Work out the finished part from the listing and answer in its coordinate system (mm). A direction names the side the tool comes from. Round coordinates to 2 decimals unless told otherwise and drop trailing zeros. Loops run counter-clockwise (first coordinate to the right, second up) from the corner with the lowest first, then second, coordinate; pieces in that order, holes last. Notation, with made-up numbers: (8.5, 74.5) - (65.5, 74.5) arc R27 cw to (65.5, 104.5) - close; hole circle Ø7 at (43, 26). An arc over 180 degrees is marked (long way). Use CSV: the item, a comma, the result in double quotes. Start each with the question number.
from build123d import *

# Parameters (mm, degrees)
EXTRUDE1_DEPTH      = 4
EXTRUDE2_DEPTH      = 12.357816692
EXTRUDE2_DEPTH_BACK = 12.357816692
SKETCH2_R           = 1
EXTRUDE3_DEPTH      = 12.357816692
EXTRUDE3_DEPTH_BACK = 12.357816692
SKETCH4_W           = 6
SKETCH4_H           = 8.732029078
FILLET1_R           = 0.2
FILLET2_R           = 1
EXTRUDE4_DEPTH      = 14
EXTRUDE4_DEPTH_BACK = 3
SKETCH3_R           = 1.5
EXTRUDE5_DEPTH      = 9
SKETCH6_R           = 1.5
EXTRUDE6_DEPTH      = 1
SKETCH7_R           = 0.6
EXTRUDE7_DEPTH      = 1
FILLET3_R           = 1
SKETCH8_R           = 2
EXTRUDE8_DEPTH      = 1
SKETCH9_W           = 5.922368331
SKETCH9_H           = 2.817570744
SKETCH9_H_2         = 4.117351233
EXTRUDE9_DEPTH      = 19.227726134


with BuildPart() as part:
    # Sketch1 → Extrude1 (new, symmetric)
    with BuildSketch(Plane.XY):
        Polygon((0, 0), (-7, 0), (-7, 8), (7, 8), (7, 0), align=None)
    extrude(amount=EXTRUDE1_DEPTH, both=True)

    # Sketch2 → Extrude2 (cut, two sides: drawn at the far end of the back side and taken through both)
    with BuildSketch(Plane.XY.offset(-EXTRUDE2_DEPTH_BACK)):
        with Locations((4.5, 4.5)):
            Circle(SKETCH2_R)
    extrude(amount=EXTRUDE2_DEPTH + EXTRUDE2_DEPTH_BACK, mode=Mode.SUBTRACT)

    # Sketch4 → Extrude3 (cut, two sides: drawn at the far end of the back side and taken through both)
    with BuildSketch(Plane(origin=(0, 0, 0), x_dir=(0, 0, -1), z_dir=(1, 0, 0)).offset(-EXTRUDE3_DEPTH_BACK)):
        with Locations((0, 5.366014539)):
            Rectangle(SKETCH4_W, SKETCH4_H)
    extrude(amount=EXTRUDE3_DEPTH + EXTRUDE3_DEPTH_BACK, mode=Mode.SUBTRACT)

    # Fillet1
    fillet1_edges = [part.edges().sort_by_distance(p)[0] for p in [
        (0, 0, 4),
        (0, 0, -4),
    ]]
    fillet(fillet1_edges, radius=FILLET1_R)

    # Fillet2
    fillet2_edges = [part.edges().sort_by_distance(p)[0] for p in [
        (-7, 8, -3.5),
        (7, 8, -3.5),
        (-7, 8, 3.5),
        (7, 8, 3.5),
    ]]
    fillet(fillet2_edges, radius=FILLET2_R)

    # Sketch3 → Extrude4 (add, two sides: drawn at the far end of the back side and taken through both)
    with BuildSketch(Plane.XY.offset(-EXTRUDE4_DEPTH_BACK)):
        with Locations((-3, 4.5)):
            Circle(SKETCH3_R)
    extrude(amount=EXTRUDE4_DEPTH + EXTRUDE4_DEPTH_BACK)

    # Sketch5 → Extrude5 (cut)
    with BuildSketch(Plane.XY.offset(14)):
        Polygon((-4, 4.5), (-4, 6.060686456), (-4.95644391, 6.060686456), (-4.95644391, 2.5), (-4, 2.5), align=None)
    extrude(amount=-EXTRUDE5_DEPTH, mode=Mode.SUBTRACT)

    # Sketch6 → Extrude6 (add)
    with BuildSketch(Plane.XZ):
        with Locations((-7, 0)):
            Circle(SKETCH6_R)
        with Locations((7, 0)):
            Circle(SKETCH6_R)
    extrude(amount=-EXTRUDE6_DEPTH)

    # Sketch7 → Extrude7 (cut)
    with BuildSketch(Plane.XZ):
        with Locations((-7, 0)):
            Circle(SKETCH7_R)
        with Locations((7, 0)):
            Circle(SKETCH7_R)
    extrude(amount=-EXTRUDE7_DEPTH, mode=Mode.SUBTRACT)

    # Fillet3
    fillet3_edges = [part.edges().sort_by_distance(p)[0] for p in [
        (7, 0.5, -1.5),
        (7, 0.5, 1.5),
        (-7, 0.5, 1.5),
        (-7, 0.5, -1.5),
    ]]
    fillet(fillet3_edges, radius=FILLET3_R)

    # Sketch8 → Extrude8 (cut)
    with BuildSketch(Plane.XZ):
        Circle(SKETCH8_R)
    extrude(amount=-EXTRUDE8_DEPTH, mode=Mode.SUBTRACT)

    # Sketch9 → Extrude9 (cut, through all)
    with BuildSketch(Plane(origin=(0, 0, 0), x_dir=(0, 0, -1), z_dir=(1, 0, 0))):
        with Locations((-12.461184166, 5.908785372)):
            Rectangle(SKETCH9_W, SKETCH9_H)
        with Locations((-12.461184166, 2.441324384)):
            Rectangle(SKETCH9_W, SKETCH9_H_2)
    extrude(amount=-EXTRUDE9_DEPTH, mode=Mode.SUBTRACT)


solid = part.part
Item 1: A cutting plane is placed at C-C (x = 4.5). Determine the outline of the cut face in (y, z).
Item 2: Which of the six approach directions +Z, -Z, +X, -X, +Y, -Y give full straight-line access (tool end or side, diameter ignored) to faces 1 (the cylindrical face through (-1.57, 4.95, 6.71)), 2 (the flat face through (-7, 3.5, -3.5)), 3 (the flat face through (7, 3.5, 3.5)), 4 (the flat face through (-7, 3.5, 3.5))?
Item 3: A cutting plane is placed at A-A (z = 0). Determine the outline of the cut face in (x, y).
Item 4: The mould has two halves that part along X. Classify faces 5 (the flat face through (-2, 0, 1)), 6 (the cylindrical face through (-0.434, 0.493, -1.952)), 7 (the cylindrical face through (-6.715, 7.699, -3.507)), 8 (the cylindrical face through (-1.57, 4.95, -0.04)): pulls with the +X half, pulls with the -X half, needs draft (parallel to the pull), parting line crosses it, or undercut.
Item 5: A cutting plane is placed at B-B (y = 0.5). Determine the outline of the cut face in (x, z), plus the area to 3 significant figures.
Item 6: Each of these flat-tipped pins is pushed along its axis until it touches: pin 1 Ø3 at (x, y) = (4.5, 4.5) entering from +Z; pin 2 Ø1.9 at (y, z) = (4, 3) entering from +X; pin 3 Ø1.9 at (y, z) = (4, 3) entering from -X. Where does it stop, or does it pass through?
Item 7: A cutting plane is placed at D-D (y = 4.5). Determine the outline of the cut face in (x, z), plus the area to 4 significant figures.
Item 8: Find the intervals of material crossed by probe 1 along Z at (x, y) = (4.5, 1.5); probe 2 along Y at (x, z) = (4.5, -3.45); probe 3 along Y at (x, z) = (-2.5, 0.75), in increasing order. Write a range as [from, to].
Result sheet:
1,outline,"(0, -3.8) arc R0.2 ccw to (0.2, -4) - (3.5, -4) - (3.5, -3) - (1, -3) - (1, 3) - (3.5, 3) - (3.5, 4) - (0.2, 4) arc R0.2 ccw to (0, 3.8) - close; (5.5, -4) - (8, -4) - (8, -3) - (5.5, -3) - close; (5.5, 3) - (8, 3) - (8, 4) - (5.5, 4) - close"
2,face 1,"+Z"
2,face 2,"-Z, -X, +Y, -Y"
2,face 3,"+Z, +X, +Y, -Y"
2,face 4,"+Z, -X, +Y, -Y"
3,outline,"(-8.5, 0) - (-7.6, 0) - (-7.6, 1) - (-8.5, 1) - close; (-6.4, 0) - (-2, 0) - (-2, 1) - (-6.4, 1) - close; circle Ø3 at (-3, 4.5); (2, 0) - (6.4, 0) - (6.4, 1) - (2, 1) - close; (7.6, 0) - (8.5, 0) - (8.5, 1) - (7.6, 1) - close"
4,face 5,"needs draft"
4,face 6,"undercut"
4,face 7,"pulls with the -X half"
4,face 8,"parting line crosses it"
5,outline,"(-7.6, -1.37) arc R1 cw to (-7, -2.29) - (-7, -4) - (7, -4) - (7, -2.29) arc R1 cw to (7.6, -1.37) arc R1.5 ccw to (7.6, 1.37) arc R1 cw to (7, 2.29) - (7, 4) - (-7, 4) - (-7, 2.29) arc R1 cw to (-7.6, 1.37) arc R1.5 ccw to start; hole circle Ø1.2 at (-7, 0); hole circle Ø4 at (0, 0); hole circle Ø1.2 at (7, 0)"
5,area,"105 mm^2"
6,pin 1,"z = 4"
6,pin 2,"x = 7"
6,pin 3,"x = -7"
7,outline,"(-7, -4) - (3.5, -4) - (3.5, -3) - (-1.5, -3) - (-1.5, 3) - (3.5, 3) - (3.5, 4) - (-1.5, 4) - (-1.5, 9.5) - (-4, 9.5) - (-4, 5) - (-4.5, 5) - (-4.5, 4) - (-7, 4) - (-7, 3) - (-4.5, 3) - (-4.5, -3) - (-7, -3) - close; (5.5, -4) - (7, -4) - (7, -3) - (5.5, -3) - close; (5.5, 3) - (7, 3) - (7, 4) - (5.5, 4) - close"
7,area,"56.25 mm^2"
8,probe 1,"[-4, -3], [3, 4]"
8,probe 2,"[0, 3.5], [5.5, 8]"
8,probe 3,"[0, 1], [3.09, 5.91]"
